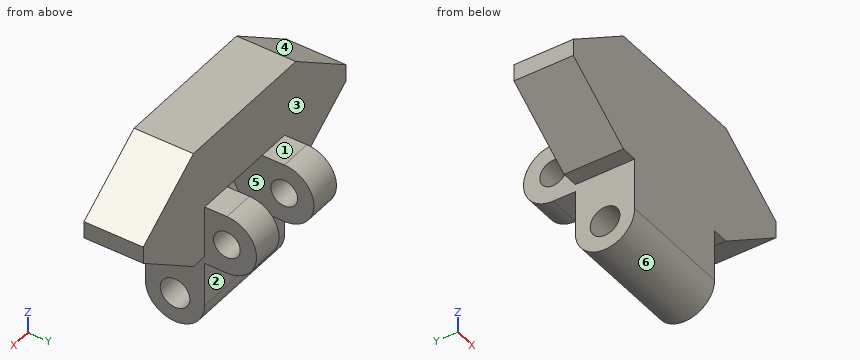
from build123d import *

# Parameters (mm, degrees)
BOSS_EXTRUDE1_DEPTH      = 4
BOSS_EXTRUDE2_DEPTH      = 3.9
BOSS_EXTRUDE2_DEPTH_BACK = 3.9
SKETCH2_R                = 1
BOSS_EXTRUDE3_DEPTH      = 3.9
BOSS_EXTRUDE3_DEPTH_BACK = 3.9
SKETCH4_R                = 0.9
CUT_EXTRUDE1_REACH       = 20.341
SKETCH5_W                = 3.4
SKETCH5_H                = 3.5
CUT_EXTRUDE2_DEPTH       = 3.4


with BuildPart() as part:
    # Sketch1 → Boss-Extrude1 (new body)
    with BuildSketch(Plane(origin=(0, 0, 0), x_dir=(1, 0, 0), z_dir=(0, 1, 0))):
        Polygon((-5, 4), (5, 4), (9.893439983, 0.573576436), (9.893439983, -0.573576436), (5, -4), (-5, -4), (-9.893439983, -0.573576436), (-9.893439983, 0.573576436), align=None)
    extrude(amount=BOSS_EXTRUDE1_DEPTH)

    # Sketch2 → Boss-Extrude2 (add, two sides: drawn at the far end of the back side and taken through both)
    with BuildSketch(Plane(origin=(0, 0, 0), x_dir=(0, 0, -1), z_dir=(1, 0, 0)).offset(-BOSS_EXTRUDE2_DEPTH_BACK)):
        with BuildLine():
            Line((4, 4), (7.5, 4))
            ThreePointArc((7.5, 4), (9.5, 2), (7.5, 0))
            Line((7.5, 0), (4, 0))
            Line((4, 0), (4, 4))
        make_face()
        with Locations((7.5, 2)):
            Circle(SKETCH2_R, mode=Mode.SUBTRACT)
    extrude(amount=BOSS_EXTRUDE2_DEPTH + BOSS_EXTRUDE2_DEPTH_BACK)

    # Sketch4 → Boss-Extrude3 (add, two sides: drawn at the far end of the back side and taken through both)
    with BuildSketch(Plane(origin=(0, 0, 0), x_dir=(0, 0, -1), z_dir=(1, 0, 0)).offset(-BOSS_EXTRUDE3_DEPTH_BACK)):
        with BuildLine():
            Line((0.5, 4), (4.5, 4))
            Line((4.5, 4), (4.5, 5.5))
            ThreePointArc((4.5, 5.5), (2.5, 7.5), (0.5, 5.5))
            Line((0.5, 5.5), (0.5, 4))
        make_face()
        with Locations((2.5, 5.5)):
            Circle(SKETCH4_R, mode=Mode.SUBTRACT)
    extrude(amount=BOSS_EXTRUDE3_DEPTH + BOSS_EXTRUDE3_DEPTH_BACK)

    # Sketch5 → Cut-Extrude1 (cut, up to next)
    with BuildSketch(Plane.XY.offset(4), mode=Mode.PRIVATE) as cut_extrude1_sk1:
        with Locations((0, 5.75)):
            Rectangle(SKETCH5_W, SKETCH5_H)
    cut_extrude1_tool1 = extrude(cut_extrude1_sk1.sketch, amount=-CUT_EXTRUDE1_REACH, mode=Mode.PRIVATE) & part.part
    add(cut_extrude1_tool1.solids().sort_by_distance((0, 5.75, 4))[0], mode=Mode.SUBTRACT)

    # Sketch6 → Cut-Extrude2 (cut)
    with BuildSketch(Plane.ZY.offset(-1.7)):
        with BuildLine():
            Line((-4.5, 4), (-0.5, 4))
            ThreePointArc((-0.5, 4), (-2.5, 2), (-4.5, 4))
        make_face()
    extrude(amount=CUT_EXTRUDE2_DEPTH, mode=Mode.SUBTRACT)


solid = part.part
Verification items for the finished model (mm, model axes). Face numbers are marked on the shaded views. A direction names the side the tool comes from. Round coordinates to 2 decimals unless told otherwise and drop trailing zeros. Write each loop counter-clockwise with the first axis right and the second up, starting at its lowest first coordinate (ties: lowest second). Pieces come first, ordered by that corner, then holes.
(1) Section check C-C (z = -2.5). Enter the section's corners in (x, y), plus the area to 3 significant figures.
Returned:
outline: (-7.14, 0) - (7.14, 0) - (7.14, 4) - (3.9, 4) - (3.9, 4.6) - (1.7, 4.6) - (1.7, 2) - (-1.7, 2) - (-1.7, 4.6) - (-3.9, 4.6) - (-3.9, 4) - (-7.14, 4) - close; (-3.9, 6.4) - (-1.7, 6.4) - (-1.7, 7.5) - (-3.9, 7.5) - close; (1.7, 6.4) - (3.9, 6.4) - (3.9, 7.5) - (1.7, 7.5) - close
area: 57.8 mm2
(2) Mould release check, pull along X, two halves, no side actions. Record for the marked faces 4, 5 and 6: pulls with the +X half, pulls with the -X half, needs draft (parallel to the pull), parting line crosses it, or undercut.
Returned:
face 4: pulls with the -X half
face 5: undercut
face 6: needs draft
(3) Depth check by flat-ended pin: pin 1 Ø0.8 at (x, y) = (3, 5) entering from +Z; pin 2 Ø3 at (y, z) = (3.5, -2.5) entering from -X; pin 3 Ø2 at (y, z) = (5.5, -2.5) entering from +X; pin 4 Ø3 at (y, z) = (2.5, 2) entering from -X. Enter the tip coordinate at first touch or a pass-through.
Returned:
pin 1: stops at z = -0.5
pin 2: stops at x = -9.28
pin 3: stops at x = 3.9
pin 4: stops at x = -9.89
(4) Access from +Z, -Z, +X, -X, +Y, -Y to the whole of each face (thin tool, end or side, straight path). Record for the marked faces 1, 2 and 3.
Returned:
face 1: +Z, +X, -X, +Y
face 2: -Z, +X, -X, +Y
face 3: +Z, +Y
(5) Section check A-A (x = 2.5). Enter the section's corners in (y, z).
Returned:
outline: (0, -7.5) arc R2 ccw to (4, -7.5) - (4, -4.5) - (5.5, -4.5) arc R2 ccw to (5.5, -0.5) - (4, -0.5) - (4, 4) - (0, 4) - close; hole circle Ø2 at (2, -7.5); hole circle Ø1.8 at (5.5, -2.5)
(6) Section check D-D (y = 7). Enter the section's corners in (x, z), plus the area to 3 significant figures.
Returned:
outline: (-3.9, -3.82) - (-1.7, -3.82) - (-1.7, -1.18) - (-3.9, -1.18) - close; (1.7, -3.82) - (3.9, -3.82) - (3.9, -1.18) - (1.7, -1.18) - close
area: 11.6 mm2
(7) Material ranges on line 1 (Y direction, x = 2, z = -7.5); line 2 (Y direction, x = -2.5, z = -2.5); line 3 (Z direction, x = 4.5, y = 3.75), recorded low to high.
Returned:
line 1: y = 0 to 1, 3 to 4
line 2: y = 0 to 4.6, 6.4 to 7.5
line 3: z = -4 to 4
(8) Section check B-B (y = 2.75). Enter the section's corners in (x, z).
Returned:
outline: (-9.89, -0.57) - (-5, -4) - (-3.9, -4) - (-3.9, -6.84) - (3.9, -6.84) - (3.9, -4) - (5, -4) - (9.89, -0.57) - (9.89, 0.57) - (5, 4) - (-5, 4) - (-9.89, 0.57) - close; (-3.9, -9.35) - (3.9, -9.35) - (3.9, -8.16) - (-3.9, -8.16) - close; hole (-1.7, -4.06) - (1.7, -4.06) - (1.7, -0.94) - (-1.7, -0.94) - close
